from build123d import *

# Parameters (mm, degrees)
SKETCH2_R           = 13.2
BOSS_EXTRUDE1_DEPTH = 2
SKETCH3_R           = 1.9
CUT_EXTRUDE1_DEPTH  = 2
SKETCH4_R           = 5
CUT_EXTRUDE2_DEPTH  = 2
CIRPATTERN1_COUNT   = 4
FILLET2_R           = 1
CUT_EXTRUDE3_START  = -10
SKETCH6_R           = 13.2
SKETCH6_R_2         = 11.4
CUT_EXTRUDE3_DEPTH  = 10


with BuildPart() as part:
    # Sketch2 → Boss-Extrude1 (new body)
    with BuildSketch(Plane(origin=(0, 0, 0), x_dir=(1, 0, 0), z_dir=(0, 1, 0))):
        with Locations(Location((0, 0, 0), (0, 0, 270))):
            Circle(SKETCH2_R)
    extrude(amount=BOSS_EXTRUDE1_DEPTH)

    # Sketch3 → Cut-Extrude1 (cut)
    with BuildSketch(Plane(origin=(0, 2, 0), x_dir=(1, 0, 0), z_dir=(0, 1, 0))):
        with Locations(Location((0, 11.2, 0), (0, 0, 270))):
            Circle(SKETCH3_R)
    cut_extrude1 = extrude(amount=-CUT_EXTRUDE1_DEPTH, mode=Mode.SUBTRACT)

    # Sketch4 → Cut-Extrude2 (cut)
    with BuildSketch(Plane(origin=(0, 2, 0), x_dir=(1, 0, 0), z_dir=(0, 1, 0))):
        with Locations(Location((0, 0, 0), (0, 0, 270))):
            Circle(SKETCH4_R)
    extrude(amount=-CUT_EXTRUDE2_DEPTH, mode=Mode.SUBTRACT)

    # CirPattern1: Cut-Extrude1 ×4 about axis
    cirpattern1_axis = Axis((0, 0, 0), (0, 1, 0))
    for i in range(1, CIRPATTERN1_COUNT):
        add(cut_extrude1.rotate(cirpattern1_axis, i * 360 / CIRPATTERN1_COUNT), mode=Mode.SUBTRACT)

    # Fillet2
    fillet2_edges = [part.edges().sort_by_distance(p)[0] for p in [
        (0, 0, -5),
        (0, 2, -5),
    ]]
    fillet(fillet2_edges, radius=FILLET2_R - 0.0001)  # a hair under: the kernel refuses the full size

    # Sketch6 → Cut-Extrude3 (cut)
    with BuildSketch(Plane(origin=(0, 2, 0), x_dir=(1, 0, 0), z_dir=(0, 1, 0)).offset(CUT_EXTRUDE3_START)):
        Circle(SKETCH6_R)
        Circle(SKETCH6_R_2, mode=Mode.SUBTRACT)
    extrude(amount=CUT_EXTRUDE3_DEPTH, mode=Mode.SUBTRACT)


solid = part.part
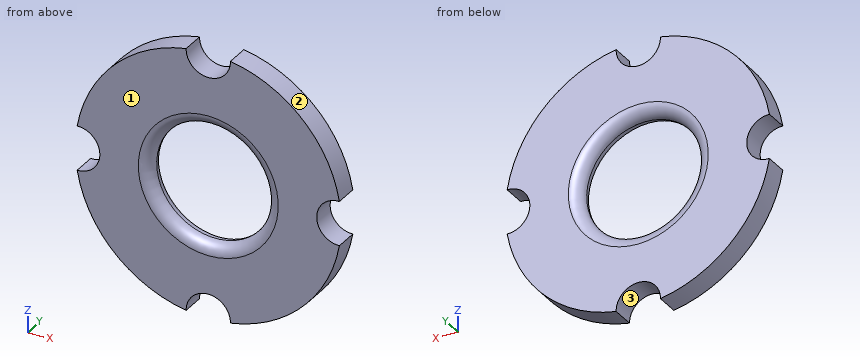
Input: part model. Units: mm. Frame: model coordinates. Face numbers are marked on the shaded views. Give positions to 0.01 mm unless a question says otherwise; leave off trailing zeros. Write each loop counter-clockwise with the first axis right and the second up, starting at its lowest first coordinate (ties: lowest second). Pieces come first, ordered by that corner, then holes. Notation, with made-up numbers: (-3.5, 5.5) -> (39.5, 5.5) arc R24 ccw to (39.5, 41.5) -> close; hole circle Ø10 at (48.25, 31). An arc over 180 degrees is marked (long way). Use one line per item in the form item = value. Start each with the question number.
1) Draft query along X for the marked faces 1, 2 and 3. Return one class per face: pulls with the +X half, pulls with the -X half, needs draft (parallel to the pull), parting line crosses it, or undercut.
2) Section query A-A on y = 1.3. Return the cut outline in (x, z), then the cut area to 3 significant figures.
3) Ray query, probe 1 along X at (y, z) = (1, 0); probe 2 along X at (y, z) = (1.45, 2.5); probe 3 along Z at (x, y) = (3.5, 0.45). Return the intervals inside material, ascending. Write a range as from..to.
4) Section query C-C on z = 8.5. Return the cut outline in (x, y), then the cut area to 3 significant figures.
5) Pin query (flat end, axial travel): pin 1 (11.5 mm diameter, centred on x = 0, z = 0, fed in from -Y). Return the tip coordinate at first contact, or that it passes through.
6) Section query B-B on z = -8. Return the cut outline in (x, y).
Outcome:
q1.face_1 = needs draft
q1.face_2 = pulls with the +X half
q1.face_3 = undercut
q2.outline = (-11.24, -1.9) arc R11.4 ccw to (-1.9, -11.24) arc R1.9 cw (long way) to (1.9, -11.24) arc R11.4 ccw to (11.24, -1.9) arc R1.9 cw (long way) to (11.24, 1.9) arc R11.4 ccw to (1.9, 11.24) arc R1.9 cw (long way) to (-1.9, 11.24) arc R11.4 ccw to (-11.24, 1.9) arc R1.9 cw (long way) to start; hole circle Ø10.09 at (0, 0)
q2.area = 303 mm^2
q3.probe_1 = -9.3..-5, 5..9.3
q3.probe_2 = -11.12..-4.45, 4.45..11.12
q3.probe_3 = -10.85..-3.8, 3.8..10.85
q4.outline = (-7.6, 0) -> (7.6, 0) -> (7.6, 2) -> (-7.6, 2) -> close
q4.area = 30.4 mm^2
q5.pin_1 = 0.03
q6.outline = (-8.12, 0) -> (8.12, 0) -> (8.12, 2) -> (-8.12, 2) -> close
